Work out the finished part from the listing and answer in its coordinate system (mm). Round coordinates to 2 decimals unless told otherwise and drop trailing zeros. Order: outer loops, then holes, each group sorted by start corner. A loop starts at its lowest first (then second) coordinate and runs counter-clockwise, first axis right, second up. Notation, with made-up numbers: (61, 64) - (70, 64) arc R21 cw to (70, 78) - close; hole circle Ø1 at (64.25, 64.5). An arc over 180 degrees is marked (long way). Answer in a Markdown table with one row per item.
Autodesk Inventor part; units mm, degrees
ref_plane "YZ Plane" through (0, 0, 0) normal (1, 0, 0) x (0, 1, 0)
ref_plane "XZ Plane" through (0, 0, 0) normal (0, 1, 0) x (-1, 0, 0)
ref_plane "XY Plane" through (0, 0, 0) normal (0, 0, 1) x (1, 0, 0)
sketch "Sketch1" plane through (0, 0, 0) normal (0, 0, 1) x (1, 0, 0)
  line L0 (-21.5, -21.5) -> (21.5, -21.5)
  line L1 (21.5, -21.5) -> (21.5, 21.5)
  line L2 (21.5, 21.5) -> (-21.5, 21.5)
  line L3 (-21.5, 21.5) -> (-21.5, -21.5)
  line L4 (-21.5, -21.5) -> (21.5, 21.5) construction
  line L5 (21.5, -21.5) -> (-21.5, 21.5) construction
  point P0 (0, 0)
  dimension "d0" = 43
  dimension "d1" = 43
extrude "Plate1" add sketch "Sketch1" along normal blind 3
chamfer "Corner Chamfer1" distance 4.5 angle 45 4 edges at (21.5, 21.5, 1.5) (-21.5, 21.5, 1.5) (-21.5, -21.5, 1.5) (21.5, -21.5, 1.5)
sketch "Sketch2" plane through (0, 0, 3) normal (0, 0, 1) x (1, 0, 0)
  line L0 (-17, 21.5) -> (17, 21.5)
  line L1 (0, 21.5) -> (0, -21.5)
  line L2 (17, -21.5) -> (-17, -21.5)
  line L3 (-21.5, -17) -> (-21.5, 17)
  line L4 (-21.5, 0) -> (21.5, 0)
  line L5 (21.5, 17) -> (21.5, -17)
  circle A0 centre (-16.75, 16.75) radius 1.6
  circle A1 centre (16.75, 16.75) radius 1.6
  circle A2 centre (-16.75, -16.75) radius 1.6
  circle A3 centre (16.75, -16.75) radius 1.6
  circle A4 centre (0, 0) radius 3.5
  dimension "d6" = 3.2
  dimension "d7" = 33.5
  dimension "d8" = 33.5
  dimension "d11" = 7
extrude "Cut1" cut sketch "Sketch2" against normal blind 3
equation "\"d9\" = Thickness"
equation "\"d2\" = Thickness"
equation "\"BendRadius\" = Thickness"
equation "\"BendReliefWidth\" = Thickness"
equation "\"BendReliefDepth\" = 0.5 * Thickness"
equation "\"CornerReliefSize\" = 4 * Thickness"
equation "\"MinimumRemnant\" = 2 * Thickness"
equation "\"TransitionRadius\" = BendRadius"
equation "\"JacobiRadiusSize\" = BendRadius"
equation "\"GapSize\" = Thickness"
properties part number "DC Motor Fixation"
1) Find section A-A, the plane y = 0. Give the vertices of the cut face in (x, z), then the cut area to 3 significant figures.
Filled in:
| item | result |
|---|---|
| outline | (-21.5, 0) - (-3.5, 0) - (-3.5, 3) - (-21.5, 3) - close; (3.5, 0) - (21.5, 0) - (21.5, 3) - (3.5, 3) - close |
| area | 108 mm^2 |
2) Each of these flat-tipped pins is pushed along its axis until it touches: pin 1 (3 mm diameter, centred on x = 16.75, y = -16.75, fed in from -Z); pin 2 (5 mm diameter, centred on x = 16.75, y = 16.75, fed in from +Z). Where does it stop, or does it pass through?
Filled in:
| item | result |
|---|---|
| pin 1 | passes through |
| pin 2 | stops at z = 3 |
3) Find the intervals of material crossed by probe 1 along Y at (x, z) = (-16.75, 2.2); probe 2 along X at (y, z) = (0, 1), in increasing order. Write a range as from..to.
Filled in:
| item | result |
|---|---|
| probe 1 | y = -21.5..-18.35, -15.15..15.15, 18.35..21.5 |
| probe 2 | x = -21.5..-3.5, 3.5..21.5 |
4) Find section C-C, the plane z = 2. Give the vertices of the cut face in (x, y).
Filled in:
| item | result |
|---|---|
| outline | (-21.5, -17) - (-17, -21.5) - (17, -21.5) - (21.5, -17) - (21.5, 17) - (17, 21.5) - (-17, 21.5) - (-21.5, 17) - close; hole circle Ø3.2 at (-16.75, -16.75); hole circle Ø3.2 at (-16.75, 16.75); hole circle Ø7 at (0, 0); hole circle Ø3.2 at (16.75, -16.75); hole circle Ø3.2 at (16.75, 16.75) |
5) The mould has two halves that part along Y. Classify faces 1 (the face through (15.57, -15.67, 1.52)), 2 (the face through (0, 21.5, 1)), 3 (the face through (4, 0, 3)): released by +Y, released by -Y, zero draft, split by the parting line, or undercut.
Filled in:
| item | result |
|---|---|
| face 1 | undercut |
| face 2 | released by +Y |
| face 3 | zero draft |
